Print and shaded views of the part. All mm, measured from the part's lowest x, y and z. A direction names the side the tool comes from. Give positions to 0.01 mm unless a question says otherwise; leave off trailing zeros. Loops run counter-clockwise (first coordinate to the right, second up) from the corner with the lowest first, then second, coordinate; pieces in that order, holes last.
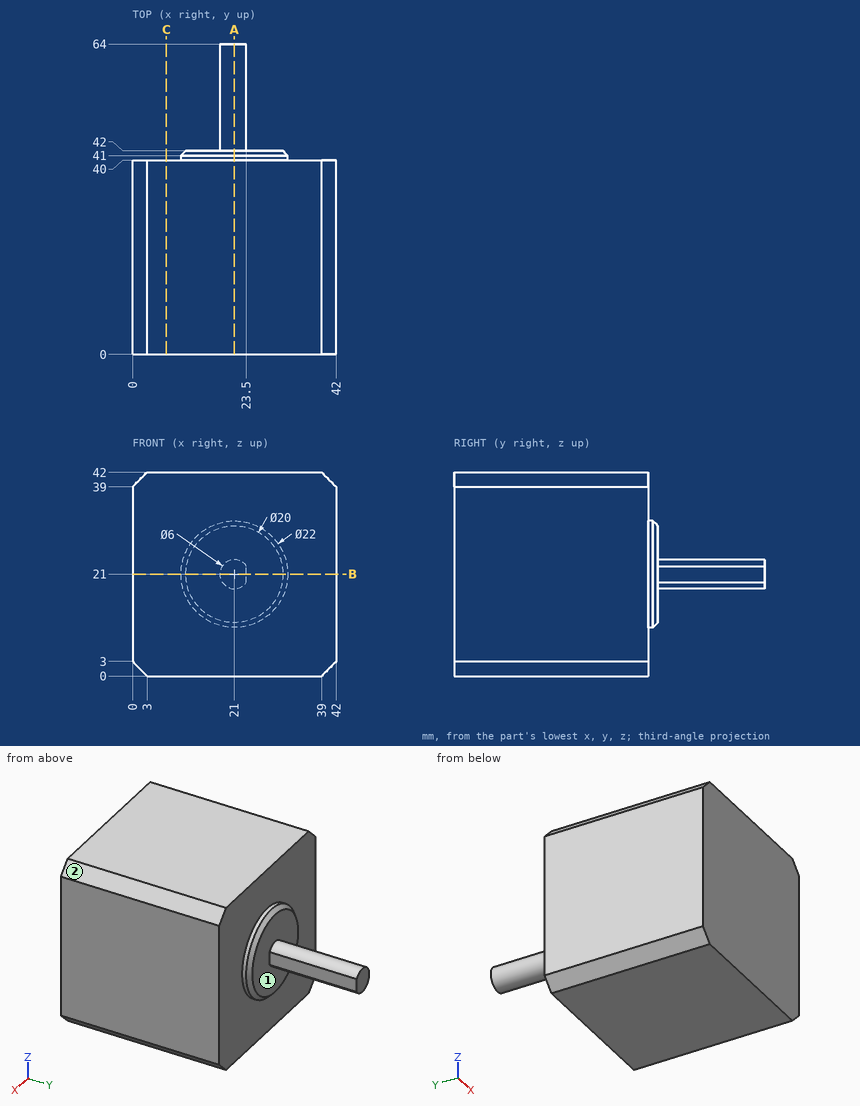
1. Tool access for the marked faces 1 and 2: list every direction of +Z, -Z, +X, -X, +Y, -Y with a clear straight run to the whole face (end or side of a thin tool).
Responses:
face 1: +Y
face 2: +Z, +X, +Y, -Y
2. Saw through at C-C, the plane x = 7. List the corners of the cut face in (y, z), and give its area (3 significant figures).
Responses:
outline: (0, 0) - (40, 0) - (40, 42) - (0, 42) - close
area: 1,680 mm2
3. Saw through at A-A, the plane x = 21. List the corners of the cut face in (y, z).
Responses:
outline: (0, 0) - (40, 0) - (40, 10) - (41, 10) - (42, 11) - (42, 18) - (64, 18) - (64, 24) - (42, 24) - (42, 31) - (41, 32) - (40, 32) - (40, 42) - (0, 42) - close
4. Probe line 1 along Y through (x, z) = (34.5, 13); line 2 along Y through (x, z) = (24, 22.5); line 3 along X through (y, z) = (61.5, 19). List the from-to ranges inside material, lowest first.
Responses:
line 1: y = 0 to 40
line 2: y = 0 to 42
line 3: x = 18.76 to 23.24
5. Drop flat-ended pins along their axis: pin 1 (5 mm diameter, centred on x = 16.5, z = 29, fed in from +Y); pin 2 (1.5 mm diameter, centred on x = 9, z = 16.5, fed in from +Y); pin 3 (1 mm diameter, centred on y = 55.5, z = 21.5, fed in from +X). Give the stop position or say it passes through.
Responses:
pin 1: stops at y = 42
pin 2: stops at y = 40
pin 3: stops at x = 23.5
6. Saw through at B-B, the plane z = 21. List the corners of the cut face in (x, y).
Responses:
outline: (0, 0) - (42, 0) - (42, 40) - (32, 40) - (32, 41) - (31, 42) - (23.5, 42) - (23.5, 64) - (18, 64) - (18, 42) - (11, 42) - (10, 41) - (10, 40) - (0, 40) - close
